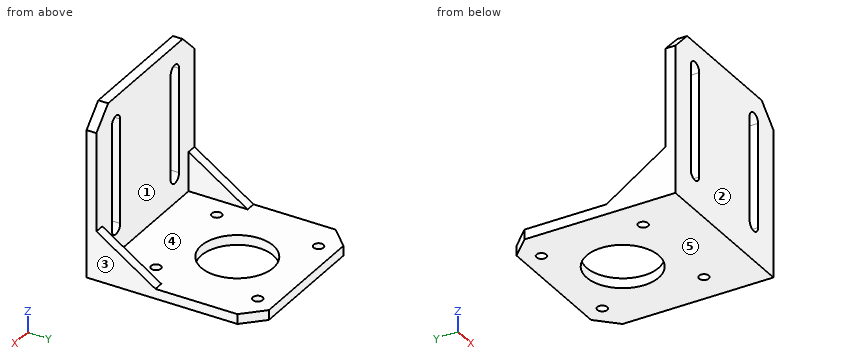
```python
from build123d import *

# Parameters (mm, degrees)
SKETCH1_R           = 11
SKETCH1_R_2         = 1.5
BOSS_EXTRUDE1_DEPTH = 3
SKETCH2_W           = 50
SKETCH2_H           = 3
BOSS_EXTRUDE2_DEPTH = 48
CUT_EXTRUDE1_REACH  = 79.006
BOSS_EXTRUDE3_START = 22
BOSS_EXTRUDE3_DEPTH = 3
LPATTERN2_COUNT     = 2
LPATTERN2_PITCH     = 47
CUT_EXTRUDE2_REACH  = 66.707
CUT_EXTRUDE3_REACH  = 79.006


with BuildPart() as part:
    # Sketch1 → Boss-Extrude1 (new body)
    with BuildSketch(Plane.XY):
        Polygon((-25, 21), (25, 21), (25, -21), (25, -31), (-25, -31), (-25, -21), align=None)
        Circle(SKETCH1_R, mode=Mode.SUBTRACT)
        with Locations((-15.5, 15.5)):
            Circle(SKETCH1_R_2, mode=Mode.SUBTRACT)
        with Locations((15.5, 15.5)):
            Circle(SKETCH1_R_2, mode=Mode.SUBTRACT)
        with Locations((-15.5, -15.5)):
            Circle(SKETCH1_R_2, mode=Mode.SUBTRACT)
        with Locations((15.5, -15.5)):
            Circle(SKETCH1_R_2, mode=Mode.SUBTRACT)
    extrude(amount=BOSS_EXTRUDE1_DEPTH)

    # Sketch2 → Boss-Extrude2 (add)
    with BuildSketch(Plane.XY.offset(3)):
        with Locations((0, -29.5)):
            Rectangle(SKETCH2_W, SKETCH2_H)
    extrude(amount=BOSS_EXTRUDE2_DEPTH)

    # Sketch3 → Cut-Extrude1 (cut, up to next)
    with BuildSketch(Plane.XZ.offset(31), mode=Mode.PRIVATE) as cut_extrude1_sk1:
        with BuildLine():
            Line((-12.85, 43), (-12.85, 11.15))
            ThreePointArc((-12.85, 11.15), (-15, 9), (-17.15, 11.15))
            Line((-17.15, 11.15), (-17.15, 43))
            ThreePointArc((-17.15, 43), (-15, 45.15), (-12.85, 43))
        make_face()
    cut_extrude1_tool1 = extrude(cut_extrude1_sk1.sketch, amount=-CUT_EXTRUDE1_REACH, mode=Mode.PRIVATE) & part.part
    # Sketch3 → Cut-Extrude1 (cut, up to next)
    with BuildSketch(Plane.XZ.offset(31), mode=Mode.PRIVATE) as cut_extrude1_sk2:
        with BuildLine():
            Line((12.85, 43), (12.85, 11.15))
            ThreePointArc((12.85, 11.15), (15, 9), (17.15, 11.15))
            Line((17.15, 11.15), (17.15, 43))
            ThreePointArc((17.15, 43), (15, 45.15), (12.85, 43))
        make_face()
    cut_extrude1_tool2 = extrude(cut_extrude1_sk2.sketch, amount=-CUT_EXTRUDE1_REACH, mode=Mode.PRIVATE) & part.part
    add(cut_extrude1_tool1.solids().sort_by_distance((-15, -31, 27.075))[0], mode=Mode.SUBTRACT)
    add(cut_extrude1_tool2.solids().sort_by_distance((15, -31, 27.075))[0], mode=Mode.SUBTRACT)

    # Sketch4 → Boss-Extrude3 (add)
    with BuildSketch(Plane(origin=(0, 0, 0), x_dir=(0, 0, -1), z_dir=(1, 0, 0)).offset(BOSS_EXTRUDE3_START)):
        Polygon((-3, -28), (-3, -10), (-15, -28), align=None)
    boss_extrude3 = extrude(amount=BOSS_EXTRUDE3_DEPTH)

    # LPattern2: Boss-Extrude3 ×2
    with Locations(*[(-i * LPATTERN2_PITCH, 0, 0) for i in range(1, LPATTERN2_COUNT)]):
        add(boss_extrude3)

    # Sketch5 → Cut-Extrude2 (cut, up to next)
    with BuildSketch(Plane(origin=(0, 0, 0), x_dir=(-1, 0, 0), z_dir=(0, 0, -1)), mode=Mode.PRIVATE) as cut_extrude2_sk1:
        Polygon((-19, 21), (-25, 15), (-25, 21), align=None)
    cut_extrude2_tool1 = extrude(cut_extrude2_sk1.sketch, amount=-CUT_EXTRUDE2_REACH, mode=Mode.PRIVATE) & part.part
    # Sketch5 → Cut-Extrude2 (cut, up to next)
    with BuildSketch(Plane(origin=(0, 0, 0), x_dir=(-1, 0, 0), z_dir=(0, 0, -1)), mode=Mode.PRIVATE) as cut_extrude2_sk2:
        Polygon((25, 21), (19, 21), (25, 15), align=None)
    cut_extrude2_tool2 = extrude(cut_extrude2_sk2.sketch, amount=-CUT_EXTRUDE2_REACH, mode=Mode.PRIVATE) & part.part
    add(cut_extrude2_tool1.solids().sort_by_distance((23, 19, 0))[0], mode=Mode.SUBTRACT)
    add(cut_extrude2_tool2.solids().sort_by_distance((-23, 19, 0))[0], mode=Mode.SUBTRACT)

    # Sketch6 → Cut-Extrude3 (cut, up to next)
    with BuildSketch(Plane.XZ.offset(31), mode=Mode.PRIVATE) as cut_extrude3_sk1:
        Polygon((-25, 51), (-25, 45), (-19, 51), align=None)
    cut_extrude3_tool1 = extrude(cut_extrude3_sk1.sketch, amount=-CUT_EXTRUDE3_REACH, mode=Mode.PRIVATE) & part.part
    # Sketch6 → Cut-Extrude3 (cut, up to next)
    with BuildSketch(Plane.XZ.offset(31), mode=Mode.PRIVATE) as cut_extrude3_sk2:
        Polygon((25, 51), (19, 51), (25, 45), align=None)
    cut_extrude3_tool2 = extrude(cut_extrude3_sk2.sketch, amount=-CUT_EXTRUDE3_REACH, mode=Mode.PRIVATE) & part.part
    add(cut_extrude3_tool1.solids().sort_by_distance((-23, -31, 49))[0], mode=Mode.SUBTRACT)
    add(cut_extrude3_tool2.solids().sort_by_distance((23, -31, 49))[0], mode=Mode.SUBTRACT)


solid = part.part
```
The listing builds one solid part. Answer for the finished solid, in the listing's coordinates (mm). Face numbers are marked on the shaded views. A direction names the side the tool comes from. Coordinates: 2 decimals unless noted, no trailing zeros. Loops run counter-clockwise (first coordinate to the right, second up) from the corner with the lowest first, then second, coordinate; pieces in that order, holes last. Notation, with made-up numbers: M 5.25,-15 L 13.25,-15 A18 ccw 13.25,16 Z; hole C -23,-6.75 d3. An arc over 180 degrees is marked long. Answer as CSV lines item,"result". Start each with the question number.
(1) Given pin 1 (6 mm diameter, centred on x = 10.5, y = 15, fed in from -Z); pin 2 (1.5 mm diameter, centred on x = 11.5, y = -8.5, fed in from +Z); pin 3 (6 mm diameter, centred on x = -7, z = 16.5, fed in from +Y); pin 4 (2.5 mm diameter, centred on x = -15.5, y = 15.5, fed in from +Z), each flat-ended and moving along its own axis, determine where each tip first touches the part or whether it passes through.
(2) The part is cut by section B-B (x = 0). Give the vertices of the cut face in (y, z), and give its area (3 significant figures).
(3) The part is cut by section D-D (x = -18). Give the vertices of the cut face in (y, z), and give its area (3 significant figures).
(4) The part is cut by section A-A (z = 23.5). Give the vertices of the cut face in (x, y).
(5) The mould has two halves that part along X. Classify the marked faces 1, 2 and 3: pulls with the +X half, pulls with the -X half, needs draft (parallel to the pull), parting line crosses it, or undercut.
(6) The part is cut by section C-C (y = 0). Give the vertices of the cut face in (x, z).
(7) Find the intervals of material crossed by L1, parallel to Y at x = -15.5, z = 2.35; L2, parallel to Y at x = 0, z = 2.2; L3, parallel to Y at x = 15, z = 1, in increasing order. Write a range as [from, to].
(8) For the marked faces 4 and 5, determine the directions among +Z, -Z, +X, -X, +Y, -Y from which every point of the face is accessible in a straight line to the end or side of a thin tool.
Determined:
1,pin 1,"z = 0"
1,pin 2,"z = 3"
1,pin 3,"y = -28"
1,pin 4,"through"
2,outline,"M -31,0 L -11,0 L -11,3 L -28,3 L -28,51 L -31,51 Z; M 11,0 L 21,0 L 21,3 L 11,3 Z"
2,area,"234 mm2"
3,outline,"M -31,0 L 21,0 L 21,3 L -28,3 L -28,51 L -31,51 Z"
3,area,"300 mm2"
4,outline,"M -25,-31 L -17.15,-31 L -17.15,-28 L -25,-28 Z; M -12.85,-31 L 12.85,-31 L 12.85,-28 L -12.85,-28 Z; M 17.15,-31 L 25,-31 L 25,-28 L 17.15,-28 Z"
5,face 1,"undercut"
5,face 2,"needs draft"
5,face 3,"pulls with the +X half"
6,outline,"M -25,0 L -11,0 L -11,3 L -25,3 Z; M 11,0 L 25,0 L 25,3 L 11,3 Z"
7,L1,"[-31, -17], [-14, 14], [17, 21]"
7,L2,"[-31, -11], [11, 21]"
7,L3,"[-31, -16.91], [-14.09, 14.09], [16.91, 21]"
8,face 4,"+Z, +Y"
8,face 5,"-Z, +X, -X, +Y, -Y"
